Autodesk Inventor part; units mm, degrees
ref_plane "YZ Plane" through (0, 0, 0) normal (1, 0, 0) x (0, 1, 0)
ref_plane "XZ Plane" through (0, 0, 0) normal (0, 1, 0) x (-1, 0, 0)
ref_plane "XY Plane" through (0, 0, 0) normal (0, 0, 1) x (1, 0, 0)
sketch "Boceto1" plane through (0, 0, 0) normal (0, 1, 0) x (-1, 0, 0)
  line L0 (0, 0) -> (3, 0)
  line L1 (3, 0) -> (3, -33)
  line L2 (3, -33) -> (0, -33)
  line L3 (0, -33) -> (0, 0)
  dimension "d0" = 3
  dimension "d1" = 33
extrude "Extrusión1" add sketch "Boceto1" along normal blind 2
sketch "Boceto2" plane through (0, 2, 0) normal (0, 1, 0) x (1, 0, 0)
  line L0 (-3, 0) -> (0, 0)
  line L1 (-1.5, 0) -> (-1.5, 10)
  line L2 (0, 33) -> (-3, 33)
  line L3 (-1.5, 33) -> (-1.5, 23)
  circle A0 centre (-1.5, 10) radius 0.95
  circle A1 centre (-1.5, 23) radius 0.95
  dimension "d4" = 10
  dimension "d5" = 10
  dimension "d8" = 1.9
  dimension "d9" = 1.9
extrude "Extrusión2" add sketch "Boceto2" along normal blind 5
sketch "Boceto3" plane through (-3, 0, -33) normal (-1, 0, 0) x (0, 0, 1)
  line L0 (0, 0) -> (33, 0)
  line L1 (33, 2) -> (0, 2)
  line L2 (33, 0) -> (0, 0)
  line L3 (0, 0) -> (0, 2)
  line L4 (0, 2) -> (33, 2)
  line L5 (33, 2) -> (33, 0)
extrude "Extrusión3" add sketch "Boceto3" along normal blind 16
properties part number "contrabase_fin_carrera"
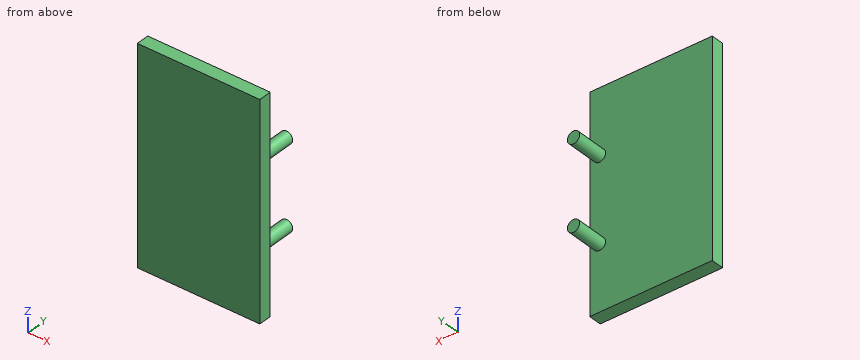
Verification items for the finished model (mm, model axes). Coordinates: 2 decimals unless noted, no trailing zeros. Loops run counter-clockwise (first coordinate to the right, second up) from the corner with the lowest first, then second, coordinate; pieces in that order, holes last. Notation, with made-up numbers: (-37, 34.25) -> (-31, 34.25) arc R33 ccw to (-31, 63.25) -> close; hole circle Ø9 at (65, 10). An arc over 180 degrees is marked (long way). Answer as a JSON object with one key per item and string values. Group by question number.
Item 1: Sectioned sample at A-A on x = -1.5. Record the boundary of the cut face in (y, z), plus the area to 3 significant figures.
Item 2: Depth check by flat-ended pin: pin 1 (5 mm diameter, centred on x = -14, z = -19.5, fed in from -Y); pin 2 (3 mm diameter, centred on x = -3.5, z = -14, fed in from +Y). Enter the tip coordinate at first touch or a pass-through.
Item 3: Sectioned sample at C-C on z = -10. Record the boundary of the cut face in (x, y).
Item 4: Sectioned sample at B-B on y = 4. Record the boundary of the cut face in (x, z), plus the area to 3 significant figures.
Item 5: Sectioned sample at D-D on z = -13.5. Record the boundary of the cut face in (x, y).
Item 6: Scan lines: probe 1 along Y at (x, z) = (-5.25, -21); probe 2 along X at (y, z) = (5.5, -23); probe 3 along Z at (x, y) = (-1, 3). Record each from-to range of solid material in increasing order.
Evaluation:
{
 "1": {"outline": "(0, -33) -> (2, -33) -> (2, -23.95) -> (7, -23.95) -> (7, -22.05) -> (2, -22.05) -> (2, -10.95) -> (7, -10.95) -> (7, -9.05) -> (2, -9.05) -> (2, 0) -> (0, 0) -> close", "area": "85.0 mm²"},
 "2": {"pin 1": "stops at y = 0", "pin 2": "stops at y = 2"},
 "3": {"outline": "(-19, 0) -> (0, 0) -> (0, 2) -> (-0.55, 2) -> (-0.55, 7) -> (-2.45, 7) -> (-2.45, 2) -> (-19, 2) -> close"},
 "4": {"outline": "circle Ø1.9 at (-1.5, -23); circle Ø1.9 at (-1.5, -10)", "area": "5.67 mm²"},
 "5": {"outline": "(-19, 0) -> (0, 0) -> (0, 2) -> (-19, 2) -> close"},
 "6": {"probe 1": "y = 0 to 2", "probe 2": "x = -2.45 to -0.55", "probe 3": "z = -23.81 to -22.19, -10.81 to -9.19"}
}
